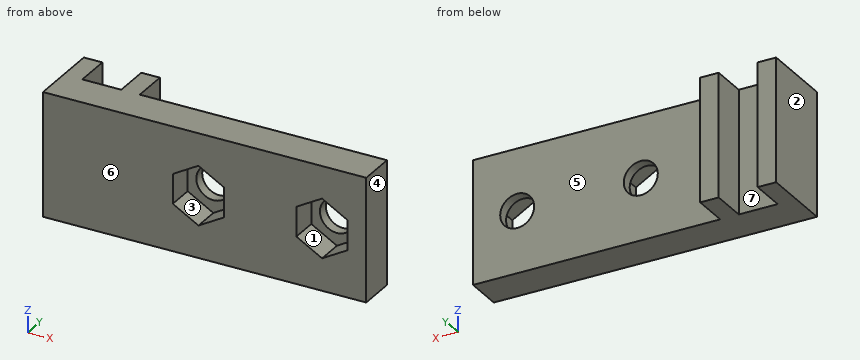
```python
from build123d import *

# Parameters (mm, degrees)
EXTRUDE_20_DEPTH         = 20
CUT_EXTRUDE_5_DEPTH      = 54.401521514
CUT_EXTRUDE_5_DEPTH_BACK = 54.401521514
SKETCH_5_R               = 2.75
CUT_EXTRUDE_5_4_3_DEPTH  = 4.3


with BuildPart() as part:
    # Профиль_скобы_6мм → Печатный_корпус_20мм (new body)
    with BuildSketch(Plane.XY):
        Polygon((-3.15, -6), (49.15, -6), (49.15, 0), (9.15, 0), (9.15, 5.8), (6.15, 5.8), (6.15, 0), (-0.15, 0), (-0.15, 5.8), (-3.15, 5.8), align=None)
    extrude(amount=EXTRUDE_20_DEPTH)

    # Sketch 5 → Винты_полки_М5 (cut, two sides: drawn at the far end of the back side and taken through both)
    with BuildSketch(Plane(origin=(0, 0, 0), x_dir=(1, 0, 0), z_dir=(0, 1, 0)).offset(-CUT_EXTRUDE_5_DEPTH_BACK)):
        with Locations(Location((22, -10, 0), (0, 0, 270))):
            Circle(SKETCH_5_R)
        with Locations(Location((42, -10, 0), (0, 0, 270))):
            Circle(SKETCH_5_R)
    extrude(amount=CUT_EXTRUDE_5_DEPTH + CUT_EXTRUDE_5_DEPTH_BACK, mode=Mode.SUBTRACT)

    # Sketch 5 2 → Гайки_полки_М5_4_3мм (cut)
    with BuildSketch(Plane.XZ.offset(6)):
        Polygon((22, 14.792007234), (26.15, 12.396003617), (26.15, 7.603996383), (22, 5.207992766), (17.85, 7.603996383), (17.85, 12.396003617), align=None)
        Polygon((42, 14.792007234), (46.15, 12.396003617), (46.15, 7.603996383), (42, 5.207992766), (37.85, 7.603996383), (37.85, 12.396003617), align=None)
    extrude(amount=-CUT_EXTRUDE_5_4_3_DEPTH, mode=Mode.SUBTRACT)


solid = part.part
```
Geometry check sheet. Reference: the model listing, model coordinates, mm. Face numbers are marked on the shaded views. A direction names the side the tool comes from. Give positions to 0.01 mm unless a question says otherwise; leave off trailing zeros. Write each loop counter-clockwise with the first axis right and the second up, starting at its lowest first coordinate (ties: lowest second). Pieces come first, ordered by that corner, then holes. Notation, with made-up numbers: (59, 47.5) -> (106, 47.5) arc R21 ccw to (106, 86.5) -> close; hole circle Ø8 at (63, 76.25). An arc over 180 degrees is marked (long way). Use one line per item in the form item = value.
Item 1: Sectioned sample at B-B on y = -0.5. Enter the section's corners in (x, z), plus the area to 3 significant figures.
Results list:
outline = (-3.15, 0) -> (49.15, 0) -> (49.15, 20) -> (-3.15, 20) -> close; hole circle Ø5.5 at (22, 10); hole circle Ø5.5 at (42, 10)
area = 998 mm2
Item 2: Access from +Z, -Z, +X, -X, +Y, -Y to the whole of each face (thin tool, end or side, straight path). Record for the marked faces 5, 6 and 7.
Results list:
face_5 = +Z, -Z, +X, +Y
face_6 = +Z, -Z, +X, -X, -Y
face_7 = +Z, -Z, +Y
Item 3: Depth check by flat-ended pin: pin 1 Ø1.7 at (y, z) = (2, 8) entering from +X; pin 2 Ø10 at (x, z) = (21.5, 7.5) entering from +Y; pin 3 Ø6.5 at (x, z) = (41.5, 10) entering from -Y. Enter the tip coordinate at first touch or a pass-through.
Results list:
pin_1 = 9.15
pin_2 = 0
pin_3 = -1.7
Item 4: Scan lines: line 1 (X direction, y = -0.9, z = 10); line 2 (X direction, y = 4, z = 14.75); line 3 (Z direction, x = 42, y = -0.6). Record each from-to range of solid material in increasing order.
Results list:
line_1 = -3.15 to 19.25, 24.75 to 39.25, 44.75 to 49.15
line_2 = -3.15 to -0.15, 6.15 to 9.15
line_3 = 0 to 7.25, 12.75 to 20
Item 5: Sectioned sample at D-D on x = 21. Enter the section's corners in (y, z).
Results list:
outline = (-6, 0) -> (0, 0) -> (0, 7.44) -> (-1.7, 7.44) -> (-1.7, 5.79) -> (-6, 5.79) -> close; (-6, 14.21) -> (-1.7, 14.21) -> (-1.7, 12.56) -> (0, 12.56) -> (0, 20) -> (-6, 20) -> close
Item 6: Sectioned sample at C-C on z = 18.75. Enter the section's corners in (x, y), plus the area to 3 significant figures.
Results list:
outline = (-3.15, -6) -> (49.15, -6) -> (49.15, 0) -> (9.15, 0) -> (9.15, 5.8) -> (6.15, 5.8) -> (6.15, 0) -> (-0.15, 0) -> (-0.15, 5.8) -> (-3.15, 5.8) -> close
area = 349 mm2
Item 7: Sectioned sample at A-A on z = 9.5. Enter the section's corners in (x, y).
Results list:
outline = (-3.15, -6) -> (17.85, -6) -> (17.85, -1.7) -> (19.3, -1.7) -> (19.3, 0) -> (9.15, 0) -> (9.15, 5.8) -> (6.15, 5.8) -> (6.15, 0) -> (-0.15, 0) -> (-0.15, 5.8) -> (-3.15, 5.8) -> close; (24.7, -1.7) -> (26.15, -1.7) -> (26.15, -6) -> (37.85, -6) -> (37.85, -1.7) -> (39.3, -1.7) -> (39.3, 0) -> (24.7, 0) -> close; (44.7, -1.7) -> (46.15, -1.7) -> (46.15, -6) -> (49.15, -6) -> (49.15, 0) -> (44.7, 0) -> close
Item 8: Mould release check, pull along X, two halves, no side actions. Record for the marked faces 1, 2, 3 and 4: released by +X, released by -X, zero draft, split by the parting line, or undercut.
Results list:
face_1 = undercut
face_2 = released by -X
face_3 = undercut
face_4 = released by +X
